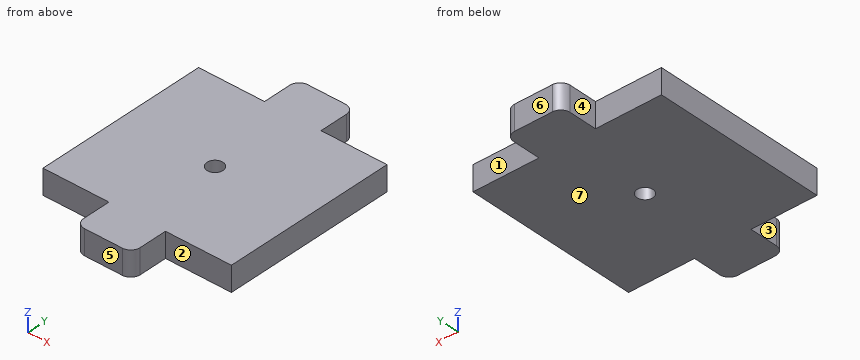
from build123d import *

# Parameters (mm, degrees)
MODEL_R             = 2.125
BOSS_EXTRUDE1_DEPTH = 6.6


with BuildPart() as part:
    # Model → Boss-Extrude1 (new body)
    with BuildSketch(Plane.XY):
        with BuildLine():
            Line((-25, 23.12), (-25, -23.12))
            Line((-25, -23.12), (-7.5, -23.12))
            Line((-7.5, -23.12), (-7.5, -30.62))
            ThreePointArc((-7.5, -30.62), (-6.767766953, -32.387766953), (-5, -33.12))
            Line((-5, -33.12), (5, -33.12))
            ThreePointArc((5, -33.12), (6.767766953, -32.387766953), (7.5, -30.62))
            Line((7.5, -30.62), (7.5, -23.12))
            Line((7.5, -23.12), (25, -23.12))
            Line((25, -23.12), (25, 23.12))
            Line((25, 23.12), (7.5, 23.12))
            Line((7.5, 23.12), (7.5, 30.62))
            ThreePointArc((7.5, 30.62), (6.767766953, 32.387766953), (5, 33.12))
            Line((5, 33.12), (-5, 33.12))
            ThreePointArc((-5, 33.12), (-6.767766953, 32.387766953), (-7.5, 30.62))
            Line((-7.5, 30.62), (-7.5, 23.12))
            Line((-7.5, 23.12), (-25, 23.12))
        make_face()
        Circle(MODEL_R, mode=Mode.SUBTRACT)
    extrude(amount=BOSS_EXTRUDE1_DEPTH)


solid = part.part
Build history of the part. All positions in model axes, mm. Face numbers are marked on the shaded views. A direction names the side the tool comes from. Round coordinates to 2 decimals unless told otherwise and drop trailing zeros. Order: outer loops, then holes, each group sorted by start corner. A loop starts at its lowest first (then second) coordinate and runs counter-clockwise, first axis right, second up. Notation, with made-up numbers: M 44,88 L 54,88 A16 cw 54,92 Z; hole C 7.5,-15 d6. An arc over 180 degrees is marked long. Use CSV: the item, a comma, the result in double quotes. Start each with the question number.
(1) Tool access for the marked faces 1, 2, 3 and 4: list every direction of +Z, -Z, +X, -X, +Y, -Y with a clear straight run to the whole face (end or side of a thin tool).
(2) Cut at D-D on x = -21. List the corners of the cut face in (y, z).
(3) Cut at B-B on x = 0. List the corners of the cut face in (y, z) (3 decimals).
(4) Flat gauge pins, fed straight in: P1, Ø3.5, axis at y = 28, z = 3.5, coming from the -X side; P2, Ø2, axis at x = 16.5, z = 3.5, coming from the -Y side; P3, Ø1.5, axis at x = -16.5, z = 4, coming from the +Y side. Where does each tip first touch, or does it go through?
(5) Mould opens along Y. For the marked faces 5, 6 and 7 say: +Y half, -Y half, draft (parallel to the pull), parting line (faces both ways), or undercut.
(6) Cut at C-C on z = 1. List the corners of the cut face in (x, y) (3 decimals).
(7) Cut at A-A on y = 0. List the corners of the cut face in (x, z) (3 decimals), then the cut area to 3 significant figures.
(8) Drill centre lines: probe 1 along Y at (x, z) = (0, 1.75) (3 decimals); probe 2 along Y at (x, z) = (-15.5, 2); probe 3 along Y at (x, z) = (-1.5, 6.5). Where is each one in solid material? Low to high.
Findings:
1,face 1,"+Z, -Z, +X, +Y"
1,face 2,"+Z, -Z, +X, -Y"
1,face 3,"+Z, -Z, -X, -Y"
1,face 4,"+Z, -Z, -X, +Y"
2,outline,"M -23.12,0 L 23.12,0 L 23.12,6.6 L -23.12,6.6 Z"
3,outline,"M -33.12,0 L -2.125,0 L -2.125,6.6 L -33.12,6.6 Z; M 2.125,0 L 33.12,0 L 33.12,6.6 L 2.125,6.6 Z"
4,P1,"stops at x = -7.5"
4,P2,"stops at y = -23.12"
4,P3,"stops at y = 23.12"
5,face 5,"-Y half"
5,face 6,"+Y half"
5,face 7,"draft"
6,outline,"M -25,-23.12 L -7.5,-23.12 L -7.5,-30.62 A2.5 ccw -5,-33.12 L 5,-33.12 A2.5 ccw 7.5,-30.62 L 7.5,-23.12 L 25,-23.12 L 25,23.12 L 7.5,23.12 L 7.5,30.62 A2.5 ccw 5,33.12 L -5,33.12 A2.5 ccw -7.5,30.62 L -7.5,23.12 L -25,23.12 Z; hole C 0,0 d4.25"
7,outline,"M -25,0 L -2.125,0 L -2.125,6.6 L -25,6.6 Z; M 2.125,0 L 25,0 L 25,6.6 L 2.125,6.6 Z"
7,area,"302 mm^2"
8,probe 1,"y = -33.12 to -2.125, 2.125 to 33.12"
8,probe 2,"y = -23.12 to 23.12"
8,probe 3,"y = -33.12 to -1.51, 1.51 to 33.12"
